```python
from build123d import *

# Parameters (mm, degrees)
CROQUIS1_R                   = 65
CROQUIS1_R_2                 = 45.25
SALIENTE_EXTRUIR1_DEPTH      = 4
TALADRO_DE_MARGEN_PARA_M31_D = 3.4
CROQUIS4_R                   = 50
CORTAR_EXTRUIR1_DEPTH        = 2


with BuildPart() as part:
    # Croquis1 → Saliente-Extruir1 (new, symmetric)
    with BuildSketch(Plane.XY):
        Circle(CROQUIS1_R)
        Circle(CROQUIS1_R_2, mode=Mode.SUBTRACT)
    extrude(amount=SALIENTE_EXTRUIR1_DEPTH, both=True)

    # Taladro de margen para M31 (through all)
    with Locations(Plane.XY.offset(4)):
        with Locations((0, 60), (42.426406871, 42.426406871), (60, 0), (42.426406871, -42.426406871), (0, -60), (-42.426406871, -42.426406871), (-60, 0), (-42.426406871, 42.426406871)):
            Hole(TALADRO_DE_MARGEN_PARA_M31_D / 2)

    # Croquis4 → Cortar-Extruir1 (cut)
    with BuildSketch(Plane(origin=(0, 0, -4), x_dir=(-1, 0, 0), z_dir=(0, 0, -1))):
        Circle(CROQUIS4_R)
    extrude(amount=-CORTAR_EXTRUIR1_DEPTH, mode=Mode.SUBTRACT)


solid = part.part
```
Geometry check sheet. Reference: the model listing, model coordinates, mm. A direction names the side the tool comes from. Coordinates: 2 decimals unless noted, no trailing zeros. Order: outer loops, then holes, each group sorted by start corner. A loop starts at its lowest first (then second) coordinate and runs counter-clockwise, first axis right, second up. Notation, with made-up numbers: M 18.5,-33 L 62.5,-33 A20 ccw 62.5,-29 Z; hole C 48,21.5 d6. An arc over 180 degrees is marked long. Answer as a JSON object with one key per item and string values.
Q1. Cross-section at C-C on x = 0. Record the cut outline in (y, z).
Results are:
{"outline": "M -65,-4 L -61.7,-4 L -61.7,4 L -65,4 Z; M -58.3,-4 L -50,-4 L -50,-2 L -45.25,-2 L -45.25,4 L -58.3,4 Z; M 45.25,-2 L 50,-2 L 50,-4 L 58.3,-4 L 58.3,4 L 45.25,4 Z; M 61.7,-4 L 65,-4 L 65,4 L 61.7,4 Z"}
Q2. Release check for a two-part mould opening along X. For faces 3 (the cylindrical face through (-41.08, 41.39, -0.06)), 4 (the flat face through (-39, -24, 4)), 5 (the cylindrical face through (62, 19.52, 0.06)) record: released by +X, released by -X, zero draft, split by the parting line, or undercut.
Results are:
{"face 3": "undercut", "face 4": "zero draft", "face 5": "split by the parting line"}
Q3. Scan lines: line 1 (Y direction, x = 0, z = -2.95); line 2 (Y direction, x = -23, z = 1.25); line 3 (Y direction, x = 21, z = 2.5). Record each from-to range of solid material in increasing order.
Results are:
{"line 1": "y = -65 to -61.7, -58.3 to -50, 50 to 58.3, 61.7 to 65", "line 2": "y = -60.79 to -38.97, 38.97 to 60.79", "line 3": "y = -61.51 to -40.08, 40.08 to 61.51"}
Q4. Depth check by flat-ended pin: pin 1 Ø2.5 at (x, y) = (42.43, -42.43) entering from +Z; pin 2 Ø1 at (y, z) = (-18.5, 2.5) entering from -X; pin 3 Ø3 at (x, z) = (-16.5, -1.5) entering from -Y; pin 4 Ø1 at (x, z) = (18.5, 0.5) entering from +Y. Enter the tip coordinate at first touch or a pass-through.
Results are:
{"pin 1": "passes through", "pin 2": "stops at x = -62.46", "pin 3": "stops at y = -63.25", "pin 4": "stops at y = 62.46"}
Q5. Tool access check on faces 1 (the flat face through (11.3, -44.2, -2)), 2 (the cylindrical face through (40.856, 41.775, -0.056)). Record the directions out of +Z, -Z, +X, -X, +Y, -Y that give a thin tool (end or side, any length) a straight path to the whole face; none if there is none.
Results are:
{"face 1": "-Z", "face 2": "+Z, -Z"}
Q6. Cross-section at A-A on x = -60. Record the cut outline in (y, z).
Results are:
{"outline": "M -25,-4 L -1.7,-4 L -1.7,4 L -25,4 Z; M 1.7,-4 L 25,-4 L 25,4 L 1.7,4 Z"}
